CAD build for the part. Positions are in the model's coordinates, mm. A direction names the side the tool comes from. Give positions to 0.01 mm unless a question says otherwise; leave off trailing zeros. Loops run counter-clockwise (first coordinate to the right, second up) from the corner with the lowest first, then second, coordinate; pieces in that order, holes last. Notation, with made-up numbers: (19.25, 78.5) - (32.25, 78.5) arc R14 ccw to (32.25, 100.5) - close; hole circle Ø3 at (85.5, -39). An arc over 180 degrees is marked (long way). Return JSON: item names as keys, results as strings.
from build123d import *

# Parameters (mm, degrees)
F0_R     = 9.525
F1_DEPTH = 38.1
F2_DEPTH = 19.05


with BuildPart() as f1:
    # F0 (on Front) → F1 (new body)
    with BuildSketch(Plane.XZ):
        Polygon((914.4, 0), (0, 914.4), (0, 0), align=None)
        with Locations((44.45, 44.45)):
            Circle(F0_R, mode=Mode.SUBTRACT)
        Polygon((699.776414305, 88.9), (88.9, 88.9), (88.9, 699.776414305), align=None, mode=Mode.SUBTRACT)
    extrude(amount=F1_DEPTH)

    # F0 (on Front) → F2 (join)
    with BuildSketch(Plane.XZ):
        Polygon((914.4, 0), (0, 914.4), (0, 0), align=None)
        with Locations((44.45, 44.45)):
            Circle(F0_R, mode=Mode.SUBTRACT)
        Polygon((699.776414305, 88.9), (88.9, 88.9), (88.9, 699.776414305), align=None, mode=Mode.SUBTRACT)
        Polygon((88.9, 699.776414305), (88.9, 88.9), (699.776414305, 88.9), align=None)
    extrude(amount=-F2_DEPTH)


solid = f1.part
1. Drill centre lines: probe 1 along Z at (x, y) = (92, -23); probe 2 along Y at (x, z) = (192.5, 141); probe 3 along Z at (x, y) = (44, 2). Where is each one in solid material? Low to high.
Values follow:
{"probe 1": "z = 0 to 88.9, 696.68 to 822.4", "probe 2": "y = 0 to 19.05", "probe 3": "z = 0 to 34.94, 53.96 to 870.4"}
2. Cut at D-D, the plane z = 783. Write the cut outline in (x, y).
Values follow:
{"outline": "(0, -38.1) - (131.4, -38.1) - (131.4, 19.05) - (0, 19.05) - close"}
3. Pull direction X, two halves, no side cores. Call faces 3 (the face through (0, -10, 464)), 4 (the face through (248, 19.05, 260)), 5 (the face through (254, 0, 263)): +X half, -X half, draft (parallel to the pull), parting line (faces both ways), or undercut.
Values follow:
{"face 3": "-X half", "face 4": "draft", "face 5": "undercut"}
4. Drop flat-ended pins along their axis: P1, Ø8, axis at x = 122, y = 1, coming from the +Z side; P2, Ø1.5, axis at y = -19, z = 190, coming from the +X side; P3, Ø1.5, axis at x = 536.5, z = 182, coming from the -Y side. Give the stop position or say it passes through.
Values follow:
{"P1": "stops at z = 796.4", "P2": "stops at x = 725.15", "P3": "stops at y = 0"}
5. Cut at A-A, the plane y = -24.5. Write the cut outline in (x, z) (3 decimals).
Values follow:
{"outline": "(0, 0) - (914.4, 0) - (0, 914.4) - close; hole circle Ø19.05 at (44.45, 44.45); hole (88.9, 88.9) - (699.776, 88.9) - (88.9, 699.776) - close"}
6. Which spindle directions (+Z, -Z, +X, -X, +Y, -Y) get a long thin tool onto all of the face, cutting with end or side? Do faces 1 (the face through (88.9, -19, 390)), 2 (the face through (387, -38.1, 425)). Say none if no direction does.
Values follow:
{"face 1": "-Y", "face 2": "+Z, -Z, +X, -X, -Y"}
7. Cut at C-C, the plane z = 433.5. Write the cut outline in (x, y).
Values follow:
{"outline": "(0, -38.1) - (88.9, -38.1) - (88.9, 0) - (355.18, 0) - (355.18, -38.1) - (480.9, -38.1) - (480.9, 19.05) - (0, 19.05) - close"}
8. Cut at B-B, the plane x = 253. Write the cut outline in (y, z).
Values follow:
{"outline": "(-38.1, 0) - (19.05, 0) - (19.05, 661.4) - (-38.1, 661.4) - (-38.1, 535.68) - (0, 535.68) - (0, 88.9) - (-38.1, 88.9) - close"}
